```python
from build123d import *

# Parameters (mm, degrees)
F0_W     = 3
F0_H     = 3
F0_H_2   = 10
F1_DEPTH = 3
F2_W     = 8
F2_H     = 80
F3_DEPTH = 25
F4_W     = 1.5
F4_H     = 10
F5_DEPTH = 25
F6_W     = 3
F6_H     = 10
F7_DEPTH = 25


with BuildPart() as f1:
    # F0 (on Top) → F1 (new body)
    with BuildSketch(Plane.XY):
        with Locations((-0.16321, -41.5)):
            Rectangle(F0_W, F0_H)
        with Locations((5.83679, -41.5)):
            Rectangle(F0_W, F0_H)
        Polygon((11.93179, 40), (-14.93179, 40), (-14.93179, -40), (-1.66321, -40), (1.33679, -40), (4.33679, -40), (7.33679, -40), (10.33679, -40), (11.93179, -40), (11.93179, -30), (11.93179, -20), (11.93179, -10), (11.93179, 0), (11.93179, 10), (11.93179, 20), (11.93179, 30), align=None)
        Polygon((11.93179, -30), (11.93179, -40), (13.33679, -40), (14.93179, -40), (14.93179, -30), align=None)
        with Locations((13.43179, -25)):
            Rectangle(F0_W, F0_H_2)
        Polygon((17.93179, -30), (14.93179, -30), (14.93179, -40), (16.52679, -40), (17.93179, -40), align=None)
        Polygon((11.93179, -40), (10.33679, -40), (10.33679, -43), (13.33679, -43), (13.33679, -40), align=None)
        with Locations((13.43179, -15)):
            Rectangle(F0_W, F0_H_2)
        with Locations((16.43179, -15)):
            Rectangle(F0_W, F0_H_2)
        with Locations((13.43179, -5)):
            Rectangle(F0_W, F0_H_2)
        with Locations((16.43179, 5)):
            Rectangle(F0_W, F0_H_2)
        with Locations((13.43179, 5)):
            Rectangle(F0_W, F0_H_2)
        with Locations((13.43179, 15)):
            Rectangle(F0_W, F0_H_2)
        with Locations((13.43179, 25)):
            Rectangle(F0_W, F0_H_2)
        with Locations((16.43179, 25)):
            Rectangle(F0_W, F0_H_2)
        with Locations((13.43179, 35)):
            Rectangle(F0_W, F0_H_2)
    extrude(amount=F1_DEPTH)

    # F2 (on face) → F3 (cut)
    with BuildSketch(Plane.XY.offset(3)):
        with Locations((-10.93179, 0)):
            Rectangle(F2_W, F2_H)
    extrude(amount=-F3_DEPTH, mode=Mode.SUBTRACT)

    # F4 (on face) → F5 (cut)
    with BuildSketch(Plane.XY.offset(3)):
        with Locations((17.18179, -35)):
            Rectangle(F4_W, F4_H)
        with Locations((17.18179, -15)):
            Rectangle(F4_W, F4_H)
    extrude(amount=-F5_DEPTH, mode=Mode.SUBTRACT)

    # F6 (on face) → F7 (cut)
    with BuildSketch(Plane.XY.offset(3)):
        with Locations((-4.53179, -10)):
            Rectangle(F6_W, F6_H)
    extrude(amount=-F7_DEPTH, mode=Mode.SUBTRACT)


solid = f1.part
```
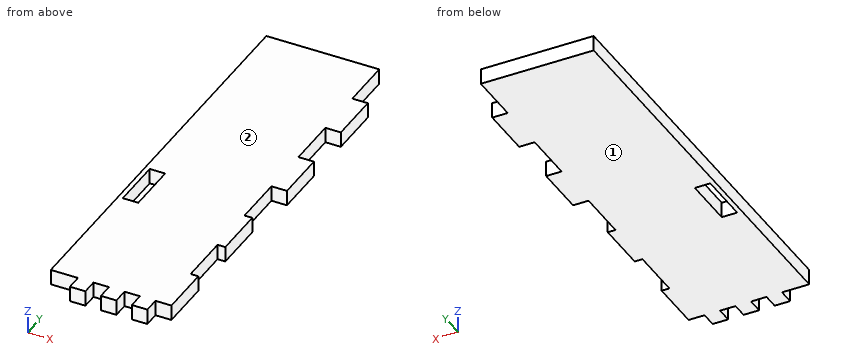
Input: part model. Units: mm. Frame: model coordinates. Face numbers are marked on the shaded views. Give positions to 0.01 mm unless a question says otherwise; leave off trailing zeros. Order: outer loops, then holes, each group sorted by start corner. A loop starts at its lowest first (then second) coordinate and runs counter-clockwise, first axis right, second up. Notation, with made-up numbers: M 67,-1 L 114,-1 A27 ccw 114,17 Z; hole C 48,30 d7. An arc over 180 degrees is marked long. One line per question, with ' | ' between items. Start each with the question number.
1. Section query A-A (x = -4.5). Return the cut outline in (y, z), and give its area (3 significant figures).
2. Section query C-C (y = -36.5). Return the cut outline in (x, z), and give its area (3 significant figures).
3. Pull-direction query (Z, two-part tool) for the marked faces 1 and 2; classes: released by +Z, released by -Z, zero draft, split by the parting line, or undercut.
4. First-contact query: pin 1 Ø0.9 at (y, z) = (-26.5, 2) entering from +X; pin 2 Ø1.5 at (y, z) = (-42, 1) entering from -X; pin 3 Ø1.5 at (x, z) = (16, 2) entering from +Y. Flat tips, straight axial feed; report the tip coordinate or a pass-through.
5. Material intervals for probe 1 along Y at (x, z) = (16, 1.2); probe 2 along Y at (x, z) = (-3.25, 0.25); probe 3 along X at (y, z) = (-13.5, 2.2), sorted ascending. Write a range as [from, to].
6. Section query D-D (y = -24). Return the cut outline in (x, z), and give its area (3 significant figures).
Here are the results:
1) outline: M -40,0 L -15,0 L -15,3 L -40,3 Z; M -5,0 L 40,0 L 40,3 L -5,3 Z | area: 210 mm²
2) outline: M -6.93,0 L 16.43,0 L 16.43,3 L -6.93,3 Z | area: 70.1 mm²
3) face 1: released by -Z | face 2: released by +Z
4) pin 1: x = 14.93 | pin 2: x = -1.66 | pin 3: y = 30
5) probe 1: [-40, -30], [-20, -10], [0, 10], [20, 30] | probe 2: [-40, -15], [-5, 40] | probe 3: [-6.93, -6.03], [-3.03, 16.43]
6) outline: M -6.93,0 L 14.93,0 L 14.93,3 L -6.93,3 Z | area: 65.6 mm²
